Autodesk Inventor part; units mm, degrees
ref_plane "Arbeitsebene1" through (0, 0, 3) normal (0, 0, -1) x (-1, 0, 0)
ref_plane "Arbeitsebene2" through (-0.6, -5.75, 3) normal (0, -1, 0) x (1, 0, 0)
ref_plane "YZ Plane" through (0, 0, 0) normal (1, 0, 0) x (0, 1, 0)
sketch "Skizze2" plane through (0, 0, 0) normal (0, 0, 1) x (1, 0, 0)
  line L0 (0, 0) -> (-0.6, 0)
  line L1 (-0.6, 0) -> (-0.6, 0.6)
  line L2 (-0.6, 0.6) -> (0, 0.6)
  line L3 (0, 0.6) -> (0, 0)
  dimension "d0" = 0.6
  dimension "d1" = 0.6
extrude "Extrusion1" add sketch "Skizze2" along normal blind 11
ref_plane "Arbeitsebene1" through (0, 0, 3) normal (0, 0, -1) x (-1, 0, 0)
sketch "Skizze3" plane through (0, 0, 3) normal (0, 0, -1) x (-1, 0, 0)
  line L0 (1.57, 1.57) -> (-0.97, 1.57)
  line L1 (-0.97, 1.57) -> (-0.97, -0.97)
  line L2 (-0.97, -0.97) -> (1.57, -0.97)
  line L3 (1.57, -0.97) -> (1.57, 1.57)
  line L4 (0.6, 0) -> (0.6, 0.6)
  line L5 (0, 0.6) -> (0.6, 0.6)
  point P0 (0, 0)
  dimension "d5" = 2.54
  dimension "d6" = 2.54
  dimension "d7" = 0.97
  dimension "d8" = 0.97
extrude "Extrusion2" add sketch "Skizze3" against normal blind 2.5
chamfer "Fase1" distance 0.25 angle 45 4 edges at (0.97, -0.97, 4.25) (-1.57, -0.97, 4.25) (-1.57, 1.57, 4.25) (0.97, 1.57, 4.25)
sketch "Skizze6" plane through (0, 0, 0) normal (0, 0, -1) x (-1, 0, 0)
  line L0 (0, 0.6) -> (0, 0)
  line L1 (0, 0.6) -> (0.6, 0.6)
  line L2 (0.6, 0.6) -> (0.6, 0)
  line L3 (0.6, 0) -> (0, 0)
  line L4 (0, 0) -> (0, 0.6)
extrude "Extrusion4" add sketch "Skizze6" along normal blind 1
sketch "Skizze7" plane through (-0.6, 0, 3) normal (0, -1, 0) x (1, 0, 0)
  line L0 (0.6, -4) -> (0, -4)
  line L1 (0.6, -4) -> (0, -4)
  line L2 (0, -4) -> (0, -3.4)
  line L3 (0, -3.4) -> (0.6, -3.4)
  line L4 (0.6, -3.4) -> (0.6, -4)
  point P0 (0.6, -3)
  dimension "d27" = 0.6
extrude "Extrusion5" add sketch "Skizze7" along normal blind 6
chamfer "Fase3" distance 0.15 angle 45 8 edges at (-0.6, 0.3, 11) (-0.3, 0, 11) (0, 0.3, 11) (-0.3, 0.6, 11) (0, -6, -0.7) (-0.3, -6, -0.4) (-0.6, -6, -0.7) (-0.3, -6, -1)
fillet "Rundung1" radius 0.8 1 edges at (-0.3, 0, -0.4)
fillet "Rundung2" radius 1.4 1 edges at (-0.3, 0.6, -1)
ref_plane "Arbeitsebene2" through (-0.6, -5.75, 3) normal (0, -1, 0) x (1, 0, 0)
sketch "Skizze8" plane through (-0.6, -5.75, 3) normal (0, -1, 0) x (1, 0, 0)
  circle A0 centre (0.3, -3.7) radius 0.325
  line L0 (0, -4) -> (0.6, -4)
  line L1 (0, -3.4) -> (0, -4)
  point P0 (0.6, -3)
  dimension "d33" = 0.65
  dimension "d34" = 0.3
  dimension "d35" = 0.3
extrude "Extrusion6" add sketch "Skizze8" against normal blind 0.5 contours A0 L0 L1 | L1 A0 | A0 L0 picked at (0.321, -3.7679)
properties part number "Stiftleiste_Male_90"
Here's how the part is built. I have some questions about the finished solid (model axes, mm). A direction names the side the tool comes from. Round coordinates to 2 decimals unless told otherwise and drop trailing zeros. Write each loop counter-clockwise with the first axis right and the second up, starting at its lowest first coordinate (ties: lowest second). Pieces come first, ordered by that corner, then holes.
Q1. If we section it at C-C on x = 0.15: Write out the boundary of the cut face in (y, z).
Q2. If we section it at B-B on z = 4: Write out the boundary of the cut face in (x, y).
Q3. Please list where these lines run through material, in increasing order: probe 1 along Y at (x, z) = (0.35, 4); probe 2 along Y at (x, z) = (-0.05, 9.5); probe 3 along Z at (x, y) = (0.7, 0).
Q4. If we section it at D-D on y = -4.25: Write out the boundary of the cut face in (x, z).
Q5. If we section it at A-A on y = -5.5: Write out the boundary of the cut face in (x, z) (3 decimals).
Q6. Will these pins go through, and if not, where does the flat tip stop? P1, Ø1.3, axis at x = 0, y = -0.5, coming from the -Z side; P2, Ø2, axis at y = -3.5, z = 0, coming from the -X side; P3, Ø0.6, axis at x = -0.5, z = 3.5, coming from the -Y side.
Q7. Which directions (+Z, -Z, +X, -X, +Y, -Y) give clear straight access to the entire face, cutting with the end or side of a thin tool? Please do faces 1 (the flat face through (0, -0.97, 4)), 2 (the cylindrical face through (-0.3, 0.2, -0.58)).
Answer below:
1. outline: (-0.97, 3) - (1.57, 3) - (1.57, 5.5) - (-0.97, 5.5) - close
2. outline: (-1.57, -0.72) - (-1.32, -0.97) - (0.72, -0.97) - (0.97, -0.72) - (0.97, 1.32) - (0.72, 1.57) - (-1.32, 1.57) - (-1.57, 1.32) - close
3. probe 1: y = -0.97 to 1.57
3. probe 2: y = 0 to 0.6
3. probe 3: z = 3 to 5.5
4. outline: (-0.6, -1) - (0, -1) - (0, -0.4) - (-0.6, -0.4) - close
5. outline: (-0.6, -1) - (-0.425, -1) arc R0.325 ccw to (-0.175, -1) - (0, -1) - (0, -0.825) arc R0.325 ccw to (0, -0.575) - (0, -0.4) - (-0.175, -0.4) arc R0.325 ccw to (-0.425, -0.4) - (-0.6, -0.4) - (-0.6, -0.575) arc R0.325 ccw to (-0.6, -0.825) - close
6. P1: stops at z = -1
6. P2: stops at x = -0.6
6. P3: stops at y = -0.97
7. face 1: +Z, +X, -X, -Y
7. face 2: -Z, +X, -X, +Y
